Model file for the job. Use its own axes, mm. A direction names the side the tool comes from. Coordinates: 2 decimals unless noted, no trailing zeros. Order: outer loops, then holes, each group sorted by start corner. A loop starts at its lowest first (then second) coordinate and runs counter-clockwise, first axis right, second up. Notation, with made-up numbers: (2.25, -27) -> (58.25, -27) arc R17 cw to (58.25, 1) -> close; hole circle Ø7 at (-26.75, 4.25). An arc over 180 degrees is marked (long way). Return JSON: item names as keys, results as strings. Group by question number.
1) Cut at C-C (y = 21.5). Write the cut outline in (x, z).
2) Flat gauge pins, fed straight in: pin 1 (5 mm diameter, centred on y = 7, z = 0.5, fed in from +X); pin 2 (3 mm diameter, centred on y = -1, z = 1, fed in from +X). Where does each tip first touch, or does it go through?
3) Which spindle directions (+Z, -Z, +X, -X, +Y, -Y) get a long thin tool onto all of the face, cutting with end or side? Do faces 1 (the flat face through (-4.4, -4.7, 2)), 2 (the cylindrical face through (-6.5, 8.5, 0.5)), 3 (the flat face through (-8.6, -4.7, 2)). Say none if no direction does.
4) Pull direction Y, two halves, no side cores. Call faces 4 (the flat face through (-5.6, -2.4, 10)), 5 (the cylindrical face through (-5.45, -1.55, 4.58)), 6 (the cylindrical face through (-8.6, -1.59, 6.56)): +Y half, -Y half, draft (parallel to the pull), parting line (faces both ways), or undercut.
5) Cut at B-B (z = 4). Write the cut outline in (x, y).
6) Probe line 1 (X direction, y = -1.5, z = 5.75); line 2 (Y direction, x = -6.5, z = 7); line 3 (X direction, y = 18.5, z = 0.75). List the from-to ranges inside material, lowest first.
7) Cut at A-A (y = 13). Write the cut outline in (x, z).
8) Cut at D-D (x = -6.5). State how many separate pieces and enclosed holes the cut face has, and give its area (3 significant figures).
Autodesk Fusion 360 part; units mm, degrees
sketch "Sketch1" plane through (0, 0, 0) normal (0, 0, 1) x (1, 0, 0)
  line L0 (-10, 25) -> (-3, 25)
  line L1 (-3, 25) -> (-3, -5)
  line L2 (-3, -5) -> (-10, -5)
  line L3 (-10, -5) -> (-10, 25)
  line L4 (-10, -5) -> (-3, 2)
  line L5 (-10, -5) -> (-0.1005, -5) construction
  line L6 (-3, -5) -> (-10, 2)
  circle A0 centre (-6.5, -1.5) radius 2
  line L7 (-10, -5) -> (-9, -5)
  line L8 (-9, -5) -> (-10, 10)
  line L9 (-3, -5) -> (-4, -5)
  line L10 (-4, -5) -> (-3, 10)
  line L11 (-10, 25) -> (-3, 18)
  line L12 (-10, 25) -> (-0.1005, 25) construction
  line L13 (-3, 25) -> (-10, 18)
  line L14 (-6.5, 25) -> (-6.5, 22)
  line L15 (-6.5, 22) -> (-6.5, 9)
  line L16 (-5, 21) -> (-8, 21)
  line L17 (-8, 21) -> (-8, 10)
  line L18 (-8, 10) -> (-5, 10)
  line L19 (-5, 10) -> (-5, 21)
  line L20 (-5, 21) -> (-8, 10) construction
  line L21 (-8, 21) -> (-5, 10) construction
  circle A1 centre (-6.5, 10) radius 1.5
  circle A2 centre (-6.5, 21) radius 1.5
  point P0 (-6.5, 15.5)
  dimension "d1" = 7
  dimension "d2" = 30
  dimension "d3" = 45
  dimension "d4" = 4
  dimension "d5" = 45
  dimension "d6" = 3
  dimension "d7" = 13
  dimension "d8" = 3
  dimension "d9" = 11
  dimension "d10" = 3
  dimension "d11" = 3
extrude "Extrude1" add sketch "Sketch1" along normal blind 2 contours L3 L11 L13 L17 A2 | L0 L11 L14 A2 | L0 L13 L14 A2 | L1 L3 L4 L6 A0 L8 L10 L11 L13 L17 L19 A1 | L1 L11 L13 L19 A2 | L4 L6 A0 L8 | L2 L4 L6 A0 L8 L10 | L4 L6 A0 L10
extrude "Extrude2" add sketch "Sketch1" along normal blind 10 contours L4 L6 A0 | L4 L6 A0 | L4 L6 A0 | L4 L6 A0
sketch "Sketch2" plane through (0, 0, 10) normal (0, 0, 1) x (-1, 0, 0)
  circle A0 centre (6.5, 1.5) radius 2
  circle A1 centre (6.5, 1.5) radius 1.05
  dimension "d16" = 2.1
extrude "Extrude3" cut sketch "Sketch2" against normal blind 13 contours A1
move_face "OffsetFaces1" offset 0.1 1 faces at (-4.5025, -1.4003, 4.6667)
fillet "Fillet1" radius 1.5 1 edges at (-8.4579, -0.7406, 2)
extrude "Extrude4" add 1 faces at (-6.5374, 24.1653, 0) along direction (0, 0, -1) blind 1
Answers below:
{
 "1": {"outline": "(-10, -1) -> (-7.91, -1) -> (-7.91, 2) -> (-10, 2) -> close; (-5.09, -1) -> (-3, -1) -> (-3, 2) -> (-5.09, 2) -> close"},
 "2": {"pin 1": "stops at x = -3.03", "pin 2": "stops at x = -3.63"},
 "3": {"face 1": "+Z, +X, -Y", "face 2": "+Z, -Z", "face 3": "+Z, -X, -Y"},
 "4": {"face 4": "draft", "face 5": "undercut", "face 6": "parting line"},
 "5": {"outline": "circle Ø4.2 at (-6.5, -1.5); hole circle Ø2.1 at (-6.5, -1.5)"},
 "6": {"line 1": "x = -8.6 to -7.55, -5.45 to -4.4", "line 2": "y = -3.6 to -2.55, -0.45 to 0.6", "line 3": "x = -10 to -8, -5 to -3"},
 "7": {"outline": "(-10, -1) -> (-8, -1) -> (-8, 2) -> (-10, 2) -> close; (-5, -1) -> (-3, -1) -> (-3, 2) -> (-5, 2) -> close"},
 "8": {"separate pieces": "3", "enclosed holes": "0", "area": "59.5 mm^2"}
}
